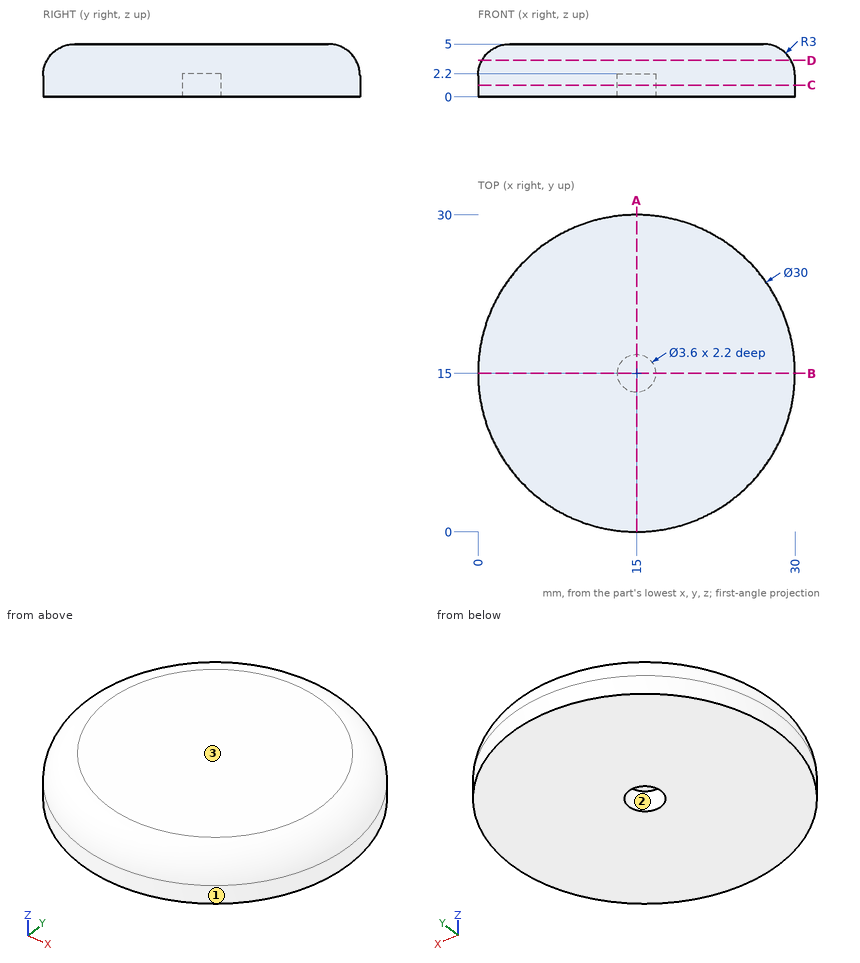
Input: dimensioned drawing with shaded views. Units: mm. Origin: part minimum x, y, z. Coordinates: 2 decimals unless noted, no trailing zeros. Order: outer loops, then holes, each group sorted by start corner. A loop starts at its lowest first (then second) coordinate and runs counter-clockwise, first axis right, second up.
(1) Material intervals for probe 1 along Y at (x, z) = (15, 1.25); probe 2 along Y at (x, z) = (14.25, 1.8); probe 3 along Y at (x, z) = (24, 2), sorted ascending.
(2) First-contact query: pin 1 (1 mm diameter, centred on x = 24.5, z = 2.5, fed in from +Y); pin 2 (1.5 mm diameter, centred on x = 6, z = 1, fed in from -Y); pin 3 (1.5 mm diameter, centred on x = 11, z = 1, fed in from +Y). Flat tips, straight axial feed; report the tip coordinate or a pass-through.
(3) Section query D-D (z = 3.45). Return the cut outline in (x, y), plus the area to 3 significant figures.
(4) Draft query along Y for the marked faces 1, 2 and 3. Return one class per face: pulls with the +Y half, pulls with the -Y half, needs draft (parallel to the pull), parting line crosses it, or undercut.
(5) Section query A-A (x = 15). Return the cut outline in (y, z), plus the area to 3 significant figures.
(6) Section query C-C (z = 1.1). Return the cut outline in (x, y), plus the area to 3 significant figures.
Solution:
1. probe 1: y = 0 to 13.2, 16.8 to 30
1. probe 2: y = 0.02 to 13.36, 16.64 to 29.98
1. probe 3: y = 3 to 27
2. pin 1: stops at y = 26.96
2. pin 2: stops at y = 2.47
2. pin 3: stops at y = 29.64
3. outline: circle Ø29.25 at (15, 15)
3. area: 672 mm2
4. face 1: parting line crosses it
4. face 2: undercut
4. face 3: needs draft
5. outline: (0, 0) - (13.2, 0) - (13.2, 2.2) - (16.8, 2.2) - (16.8, 0) - (30, 0) - (30, 2) arc R3 ccw to (27, 5) - (3, 5) arc R3 ccw to (0, 2) - close
5. area: 138 mm2
6. outline: circle Ø30 at (15, 15); hole circle Ø3.6 at (15, 15)
6. area: 697 mm2
